Source: CAD feature listing. Evaluate the final solid. Frame: model axes, mm. Face numbers are marked on the shaded views. A direction names the side the tool comes from. Round coordinates to 2 decimals unless told otherwise and drop trailing zeros. Order: outer loops, then holes, each group sorted by start corner. A loop starts at its lowest first (then second) coordinate and runs counter-clockwise, first axis right, second up.
Autodesk Inventor part; units mm, degrees
ref_plane "YZ Plane" through (0, 0, 0) normal (1, 0, 0) x (0, 1, 0)
ref_plane "XZ Plane" through (0, 0, 0) normal (0, 1, 0) x (-1, 0, 0)
ref_plane "XY Plane" through (0, 0, 0) normal (0, 0, 1) x (1, 0, 0)
sketch "Sketch1" plane through (0, 0, 0) normal (0, 0, 1) x (1, 0, 0)
  line L0 (-14.985, -7.62) -> (14.985, -7.62)
  line L1 (14.985, -7.62) -> (14.985, 7.62)
  line L2 (14.985, 7.62) -> (-14.985, 7.62)
  line L3 (-14.985, 7.62) -> (-14.985, -7.62)
  line L4 (-14.985, -7.62) -> (14.985, 7.62) construction
  line L5 (14.985, -7.62) -> (-14.985, 7.62) construction
  circle A0 centre (-13.715, 6.35) radius 0.5
  circle A1 centre (-13.715, 3.81) radius 0.5
  circle A2 centre (-13.715, 1.27) radius 0.5
  circle A3 centre (-13.715, -1.27) radius 0.5
  circle A4 centre (-13.715, -3.81) radius 0.5
  circle A5 centre (-13.715, -6.35) radius 0.5
  circle A6 centre (13.975, 6.35) radius 0.3
  circle A7 centre (13.975, -6.35) radius 0.3
  point P0 (0, 0)
  dimension "d0" = 29.97
  dimension "d1" = 15.24
  dimension "d2" = 1
  dimension "d3" = 1.27
  dimension "d4" = 1.27
  dimension "d7" = 2.54
  dimension "d12" = 0.6
  dimension "d13" = 28.96
extrude "Extrusion1" add sketch "Sketch1" along normal mid plane 0.79
sketch "Sketch2" plane through (0, 0, -0.395) normal (0, 0, -1) x (-1, 0, 0)
  circle A0 centre (13.715, -6.35) radius 0.5
  circle A1 centre (13.715, -3.81) radius 0.5
  circle A2 centre (13.715, -1.27) radius 0.5
  circle A3 centre (13.715, 1.27) radius 0.5
  circle A4 centre (13.715, 3.81) radius 0.5
  circle A5 centre (13.715, 6.35) radius 0.5
  circle A6 centre (-13.975, -6.35) radius 0.3
  circle A7 centre (-13.975, 6.35) radius 0.3
  line L0 (-14.985, -7.62) -> (14.985, -7.62)
  line L1 (14.985, -7.62) -> (14.985, 7.62)
  line L2 (14.985, 7.62) -> (-14.985, 7.62)
  line L3 (-14.985, 7.62) -> (-14.985, -7.62)
  line L4 (-13.485, 7) -> (10.985, 7)
  line L5 (10.985, 7) -> (10.985, -7)
  line L6 (10.985, -7) -> (-13.485, -7)
  line L7 (-13.485, -7) -> (-13.485, 7)
  point P0 (0, 0)
  point P1 (10.985, 0)
  dimension "d16" = 14
  dimension "d17" = 4
  dimension "d18" = 1.5
extrude "Extrusion2" add sketch "Sketch2" along normal blind 1.95 contours L4 L5 L6 L7
sketch "Sketch3" plane through (0, 0, 0.395) normal (0, 0, 1) x (1, 0, 0)
  circle A0 centre (-13.715, -6.35) radius 0.5
  circle A1 centre (-13.715, -3.81) radius 0.5
  circle A2 centre (-13.715, -1.27) radius 0.5
  circle A3 centre (-13.715, 1.27) radius 0.5
  circle A4 centre (-13.715, 3.81) radius 0.5
  circle A5 centre (-13.715, 6.35) radius 0.5
  circle A6 centre (13.975, -6.35) radius 0.3
  circle A7 centre (13.975, 6.35) radius 0.3
  line L0 (-14.985, -7.62) -> (14.985, -7.62)
  line L1 (14.985, -7.62) -> (14.985, 7.62)
  line L2 (14.985, 7.62) -> (-14.985, 7.62)
  line L3 (-14.985, 7.62) -> (-14.985, -7.62)
  line L4 (-14.985, 7.5559) -> (14.985, 7.5559) construction
  line L5 (14.985, 7.5559) -> (14.985, -7.62) construction
  line L6 (14.985, -7.62) -> (-14.985, -7.62) construction
  line L7 (-14.985, -7.62) -> (-14.985, 7.5559) construction
  line L8 (-14.985, 7.62) -> (-14.985, -7.62)
  arc A8 (13.285, 3.0475) -> (13.7564, 1.9557) centre (14.785, 3.0475) ccw
  arc A9 (13.5911, -1.0954) -> (13.7564, 1.9557) centre (12.385, 0.5) ccw
  arc A10 (13.5911, -1.0954) -> (13.032, -2.6201) centre (14.4957, -2.292) ccw
  arc A11 (5.9038, -6.579) -> (13.032, -2.6201) centre (8.885, -3.55) ccw
  arc A12 (5.9038, -6.579) -> (4.3962, -6.0072) centre (4.5009, -8.0044) ccw
  line L9 (4.3962, -6.0072) -> (-5.0076, -6.5)
  arc A13 (-6.7728, -5.8952) -> (-5.0076, -6.5) centre (-5.1385, -4.0034) ccw
  arc A14 (-6.7728, -5.8952) -> (-7.6381, -5.9802) centre (-7.165, -6.3493) ccw
  arc A15 (-10.454, -3.18) -> (-7.6381, -5.9802) centre (-9.215, -4.75) ccw
  arc A16 (-10.454, -3.18) -> (-10.454, -2.395) centre (-10.7637, -2.7875) ccw
  arc A17 (-11.215, -0.825) -> (-10.454, -2.395) centre (-9.215, -0.825) ccw
  line L10 (-11.215, -0.825) -> (-11.215, 1.675)
  arc A18 (-10.454, 3.245) -> (-11.215, 1.675) centre (-9.215, 1.675) ccw
  arc A19 (-10.454, 3.245) -> (-10.454, 4.03) centre (-10.7637, 3.6375) ccw
  arc A20 (-7.6381, 6.8302) -> (-10.454, 4.03) centre (-9.215, 5.6) ccw
  arc A21 (-7.6381, 6.8302) -> (-6.6908, 6.8317) centre (-7.165, 7.1993) ccw
  line L11 (13.285, 3.0475) -> (13.285, 5.3)
  arc A22 (13.285, 5.3) -> (10.785, 7.8) centre (10.785, 5.3) ccw
  line L12 (10.785, 7.8) -> (-4.715, 7.8)
  arc A23 (-4.715, 7.8) -> (-6.6908, 6.8317) centre (-4.715, 5.3) ccw
  circle A24 centre (-9.215, 5.6) radius 0.5
  circle A25 centre (-9.215, -4.75) radius 0.5
  circle A26 centre (12.385, 0.5) radius 0.5
  line L13 (8.885, -7.8) -> (8.885, 7.8) construction
  point P0 (0, 0)
  point P1 (8.885, 0)
  dimension "d29" = 7.8
  dimension "d32" = 4.5
  dimension "d33" = 2.5
  dimension "d34" = 26.1
  dimension "d35" = 24.5
  dimension "d36" = 5.6
  dimension "d37" = 4.75
  dimension "d38" = 2
  dimension "d44" = 2.5
  dimension "d46" = 0.5
  dimension "d49" = 2
  dimension "d52" = 0.6
  dimension "d53" = 2.5
  dimension "d54" = 4.5
  dimension "d57" = 2.5
  dimension "d59" = 0.5
  dimension "d61" = 2
  dimension "d64" = 1.5
  dimension "d65" = 1
  dimension "d73" = 20.1
  dimension "d77" = 4.25
  dimension "d78" = 3
  dimension "d80" = 2.5
  dimension "d82" = 6.5
  dimension "d84" = 2
extrude "Extrusion3" add sketch "Sketch3" along normal blind 5.87 contours A11 A12 L9 A13 A14 A15 A16 A17 L10 A18 A19 A20 A21 A23 L2 A22 L11 A8 A9 A10 L0 | L0 A11 | A23 L12 A22 L2
equation "\"d4\" = d3"
properties part number "66-0008" material "ABS Plastic"
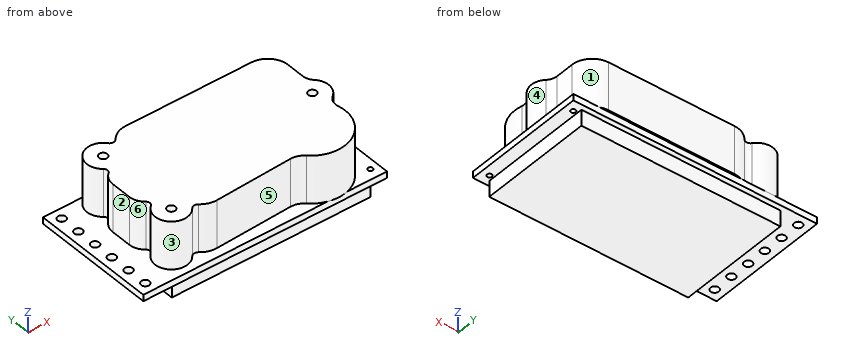
1. Section B-B on x = 8. Return loops of the section in (y, z) (3 decimals).
2. First-contact query: pin 1 (0.6 mm diameter, centred on x = -4.5, z = -1.5, fed in from +Y); pin 2 (0.6 mm diameter, centred on y = -2, z = -1, fed in from +X) (3 decimals); pin 3 (3 mm diameter, centred on y = 0.5, z = 3, fed in from -X) (3 decimals); pin 4 (5 mm diameter, centred on x = 11.5, z = 2, fed in from -Y). Flat tips, straight axial feed; report the tip coordinate or a pass-through.
3. Pull-direction query (Y, two-part tool) for the marked faces 4, 5 and 6; classes: released by +Y, released by -Y, zero draft, split by the parting line, or undercut.
4. Section C-C on y = -3.81. Return loops of the section in (x, z) (3 decimals).
5. Section A-A on y = 2.75. Return loops of the section in (x, z) (3 decimals).
6. Section D-D on z = 1. State how many separate pieces and enclosed holes the cut face has, plus the area to 3 significant figures.
7. Line query: line 1 along Z through (x, y) = (-12.75, -5.5) (3 decimals); line 2 along Y through (x, z) = (3.5, 0); line 3 along X through (y, z) = (6.75, 2.5). Output: solid intervals per line, ascending.
8. Access query for the marked faces 1, 2 and 3. Directions: +Z, -Z, +X, -X, +Y, -Y. A direction counts if a zero-diameter tool reaches every point of the face in a straight line with its end or side. Return the directions, or none.
Result:
1. outline: (-7.707, 0.395) - (-7.62, 0.395) - (-7.62, -0.395) - (-7, -0.395) - (-7, -2.345) - (7, -2.345) - (7, -0.395) - (7.62, -0.395) - (7.62, 0.395) - (7.8, 0.395) - (7.8, 6.265) - (-7.707, 6.265) - close
2. pin 1: stops at y = 7
2. pin 2: stops at x = 13.485
2. pin 3: stops at x = -11.215
2. pin 4: stops at y = -7.8
3. face 4: split by the parting line
3. face 5: released by -Y
3. face 6: undercut
4. outline: (-14.985, -0.395) - (-14.215, -0.395) - (-14.215, 0.395) - (-14.985, 0.395) - close; (-13.215, -0.395) - (-10.985, -0.395) - (-10.985, -2.345) - (13.485, -2.345) - (13.485, -0.395) - (14.985, -0.395) - (14.985, 0.395) - (13.127, 0.395) - (13.127, 6.265) - (-10.98, 6.265) - (-10.98, 0.395) - (-13.215, 0.395) - close
5. outline: (-14.985, -0.395) - (-10.985, -0.395) - (-10.985, -2.345) - (13.485, -2.345) - (13.485, -0.395) - (14.985, -0.395) - (14.985, 0.395) - (13.315, 0.395) - (13.315, 6.265) - (-10.902, 6.265) - (-10.902, 0.395) - (-14.985, 0.395) - close
6. separate pieces: 1
6. enclosed holes: 3
6. area: 343 mm2
7. line 1: z = -0.395 to 0.395
7. line 2: y = -7.62 to 7.62
7. line 3: x = -10.85 to -7.56, -6.77 to 12.82
8. face 1: +Z, +X, +Y
8. face 2: +Z, -X, +Y, -Y
8. face 3: +Z
